Read the model definition and answer for the solid it produces. Units are mm, in the model's axes. A direction names the side the tool comes from. Coordinates: 2 decimals unless noted, no trailing zeros. Loops run counter-clockwise (first coordinate to the right, second up) from the corner with the lowest first, then second, coordinate; pieces in that order, holes last. Notation, with made-up numbers: (-14, 74.25) - (24, 74.25) arc R33 cw to (24, 108.25) - close; hole circle Ø10 at (-12, 71). An arc over 180 degrees is marked (long way). One line per item, written item: value. Start each with the question number.
from build123d import *

# Parameters (mm, degrees)
BOSS_EXTRUDE1_DEPTH = 7.5
FILLET1_R           = 5
SKETCH4_W           = 15
SKETCH4_H           = 20
CUT_EXTRUDE1_DEPTH  = 152.492574085
CUT_EXTRUDE2_DEPTH  = 152.848641751
BOSS_EXTRUDE2_DEPTH = 80
BOSS_EXTRUDE3_START = 5
BOSS_EXTRUDE3_DEPTH = 5
SKETCH9_W           = 12.5
SKETCH9_H           = 20
CUT_EXTRUDE3_DEPTH  = 3
SKETCH10_W          = 2.5
SKETCH10_H          = 200
CUT_EXTRUDE4_DEPTH  = 175.180940404
SKETCH11_R          = 1.85
CUT_EXTRUDE5_DEPTH  = 167.580310961
SKETCH12_R          = 3
SKETCH12_R_2        = 3.25
CUT_EXTRUDE6_DEPTH  = 1
CUT_EXTRUDE7_DEPTH  = 7.5


with BuildPart() as part:
    # Sketch1 → Boss-Extrude1 (new, symmetric)
    with BuildSketch(Plane.XY):
        with BuildLine():
            Line((-7.4, -150), (7.4, -150))
            Line((7.4, -150), (7.4, -100))
            Line((7.4, -100), (15, -100))
            Line((15, -100), (15, 100))
            ThreePointArc((15, 100), (0, 115), (-15, 100))
            Line((-15, 100), (-15, -100))
            Line((-15, -100), (-7.4, -100))
            Line((-7.4, -100), (-7.4, -150))
        make_face()
    extrude(amount=BOSS_EXTRUDE1_DEPTH, both=True)

    # Fillet1
    fillet1_edges = [part.edges().sort_by_distance(p)[0] for p in [
        (7.4, -150, 0),
        (-7.4, -150, 0),
        (15, 0, 7.5),
        (0, 115, 7.5),
        (-15, 0, 7.5),
        (-15, 0, -7.5),
        (0, 115, -7.5),
        (15, 0, -7.5),
    ]]
    fillet(fillet1_edges, radius=FILLET1_R)

    # Sketch4 → Cut-Extrude1 (cut, through all)
    with BuildSketch(Plane.XY.offset(7.5)):
        with Locations((0, -10)):
            Rectangle(SKETCH4_W, SKETCH4_H)
    extrude(amount=-CUT_EXTRUDE1_DEPTH, mode=Mode.SUBTRACT)

    # Sketch5 → Revolve2 (revolve)
    with BuildSketch(Plane.XY):
        with BuildLine():
            Line((-7.5, -10), (-5.5, -10))
            ThreePointArc((-5.5, -10), (-6.085786438, -8.585786438), (-7.5, -8))
            Line((-7.5, -8), (-7.5, -10))
        make_face()
        with BuildLine():
            Line((7.5, -10), (5.5, -10))
            ThreePointArc((5.5, -10), (6.085786438, -8.585786438), (7.5, -8))
            Line((7.5, -8), (7.5, -10))
        make_face()
    revolve(axis=Axis((-21.965922243, -10, 0), (1, 0, 0)))

    # Sketch2 → Cut-Revolve1 (revolve, cut)
    with BuildSketch(Plane.XY):
        with BuildLine():
            Line((-7.4, -138), (-7.4, -140))
            Line((-7.4, -140), (-5.4, -140))
            ThreePointArc((-5.4, -140), (-5.985786438, -138.585786438), (-7.4, -138))
        make_face()
        with BuildLine():
            Line((7.4, -138), (7.4, -140))
            Line((7.4, -140), (5.4, -140))
            ThreePointArc((5.4, -140), (5.985786438, -138.585786438), (7.4, -138))
        make_face()
    revolve(axis=Axis((-23.291382295, -140, 0), (1, 0, 0)), mode=Mode.SUBTRACT)

    # Sketch6 → Cut-Extrude2 (cut, through all)
    with BuildSketch(Plane.ZY.offset(7.4)):
        with BuildLine():
            Line((-7.5, -137.5), (-7.5, -150))
            Line((-7.5, -150), (7.5, -150))
            Line((7.5, -150), (7.5, -137.5))
            ThreePointArc((7.5, -137.5), (0, -145), (-7.5, -137.5))
        make_face()
    extrude(amount=-CUT_EXTRUDE2_DEPTH, mode=Mode.SUBTRACT)

    # Sketch3 → Boss-Extrude2 (add)
    with BuildSketch(Plane(origin=(0, 0, 0), x_dir=(0, 0, -1), z_dir=(1, 0, 0))):
        with BuildLine():
            Line((17, -109.987492178), (17, -104.987492178))
            ThreePointArc((17, -104.987492178), (12.403805922, -103.083686255), (10.5, -98.487492178))
            Line((10.5, -98.487492178), (10.5, 100))
            Line((10.5, 100), (7.5, 100))
            Line((7.5, 100), (7.5, -100))
            ThreePointArc((7.5, -100), (10.254311627, -106.892024376), (17, -109.987492178))
        make_face()
    extrude(amount=BOSS_EXTRUDE2_DEPTH)

    # Sketch7 → Boss-Extrude3 (add)
    with BuildSketch(Plane.ZY.offset(BOSS_EXTRUDE3_START)):
        with BuildLine():
            Line((-10.5, 100), (-7.5, 100))
            Line((-7.5, 100), (-7.5, 0))
            Line((-7.5, 0), (-7.5, -20))
            Line((-7.5, -20), (-7.5, -100))
            ThreePointArc((-7.5, -100), (-10.254311627, -106.892024376), (-17, -109.987492178))
            Line((-17, -109.987492178), (-17, -104.987492178))
            ThreePointArc((-17, -104.987492178), (-12.403805922, -103.083686255), (-10.5, -98.487492178))
            Line((-10.5, -98.487492178), (-10.5, 100))
        make_face()
    extrude(amount=-BOSS_EXTRUDE3_DEPTH)

    # Sketch9 → Cut-Extrude3 (cut)
    with BuildSketch(Plane(origin=(0, 0, -10.5), x_dir=(-1, 0, 0), z_dir=(0, 0, -1))):
        with Locations((-1.25, -10)):
            Rectangle(SKETCH9_W, SKETCH9_H)
    extrude(amount=-CUT_EXTRUDE3_DEPTH, mode=Mode.SUBTRACT)

    # Sketch10 → Cut-Extrude4 (cut, through all)
    with BuildSketch(Plane.ZY.offset(15)):
        with Locations((6.25, 0)):
            Rectangle(SKETCH10_W, SKETCH10_H)
    extrude(amount=-CUT_EXTRUDE4_DEPTH, mode=Mode.SUBTRACT)

    # Sketch11 → Cut-Extrude5 (cut, through all)
    with BuildSketch(Plane(origin=(0, 0, -10.5), x_dir=(-1, 0, 0), z_dir=(0, 0, -1))):
        with Locations(Location((-38, 83.512507822, 0), (0, 0, 90))):
            Circle(SKETCH11_R)
        with Locations(Location((-38, 51.512507822, 0), (0, 0, 90))):
            Circle(SKETCH11_R)
        with Locations(Location((-70, 83.512507822, 0), (0, 0, 90))):
            Circle(SKETCH11_R)
        with Locations(Location((-70, 51.512507822, 0), (0, 0, 90))):
            Circle(SKETCH11_R)
        Polygon((-46.5, 87.012507822), (-61.5, 87.012507822), (-73.5, 75.012507822), (-73.5, 60.012507822), (-61.5, 48.012507822), (-46.5, 48.012507822), (-34.5, 60.012507822), (-34.5, 75.012507822), align=None)
    extrude(amount=-CUT_EXTRUDE5_DEPTH, mode=Mode.SUBTRACT)

    # Sketch12 → Cut-Extrude6 (cut)
    with BuildSketch(Plane(origin=(0, 0, -10.5), x_dir=(-1, 0, 0), z_dir=(0, 0, -1))):
        with Locations(Location((-38, 83.512507822, 0), (0, 0, 90))):
            Circle(SKETCH12_R)
        with Locations(Location((-70, 83.512507822, 0), (0, 0, 90))):
            Circle(SKETCH12_R)
        with Locations(Location((-70, 51.512507822, 0), (0, 0, 90))):
            Circle(SKETCH12_R)
        with Locations(Location((-38, 51.512507822, 0), (0, 0, 90))):
            Circle(SKETCH12_R_2)
    extrude(amount=-CUT_EXTRUDE6_DEPTH, mode=Mode.SUBTRACT)

    # Sketch13 → Cut-Extrude7 (cut, symmetric)
    with BuildSketch(Plane(origin=(0, 0, 0), x_dir=(0, 0, -1), z_dir=(1, 0, 0))):
        Polygon((2.75, 0), (-5, 0), (-5, 12), align=None)
    extrude(amount=CUT_EXTRUDE7_DEPTH, both=True, mode=Mode.SUBTRACT)


solid = part.part
1) Section B-B, the plane y = -94.5 is taken. Determine the outline of the cut face in (x, z), and give its area (3 significant figures).
2) Section A-A, the plane x = 0 is taken. Determine the outline of the cut face in (y, z), and give its area (3 significant figures).
3) Straight lines are drawn through the part: L1, parallel to Z at x = 14, y = 25; L2, parallel to X at y = -46.5, z = -2.5; L3, parallel to Z at x = 26.5, y = -52.5. For each, find the intervals that lie inside material, in ascending order.
4) Section C-C, the plane x = 30.5 is taken. Determine the outline of the cut face in (y, z).
5) Determine the mould class of faces 6 (the flat face through (0, 104, 7.5)), 7 (the cylindrical face through (-13.57, -1.4, -6)), 8 (the flat face through (7.4, -123, 0)), 9 (the flat face through (-7.5, -8, -1)) for opening direction X: released by +X, released by -X, zero draft, split by the parting line, or undercut.
6) Flat-ended cylindrical pins translate along their axes: P1, Ø4, axis at y = 51, z = -3, coming from the +X side; P2, Ø2, axis at x = 15, z = -11.5, coming from the -Y side; P3, Ø3.5, axis at x = 25.5, z = -9, coming from the +Y side; P4, Ø2, axis at x = 38, y = 51.51, coming from the +Z side. Find the tip coordinate at first contact, or state that the pin passes through.
7) For faces 1 (the flat face through (15, -1, 0)), 2 (the flat face through (11, -100, -1)), 3 (the flat face through (0, -20, -3)), 4 (the cylindrical face through (68.175, 81.132, -10.007)), 5 (the flat face through (-5, -65, -8)), determine the directions among +Z, -Z, +X, -X, +Y, -Y from which every point of the face is accessible in a straight line to the end or side of a thin tool.
Answer below:
1. outline: (-15, -2.5) arc R5 ccw to (-10, -7.5) - (-5, -7.5) - (-5, -10.5) - (80, -10.5) - (80, -7.5) - (10, -7.5) arc R5 ccw to (15, -2.5) - (15, 2.5) arc R5 ccw to (14.33, 5) - (-14.33, 5) arc R5 ccw to (-15, 2.5) - close
1. area: 618 mm2
2. outline: (-137.5, -7.5) - (-100, -7.5) arc R10 ccw to (-109.99, -17) - (-104.99, -17) arc R6.5 cw to (-98.49, -10.5) - (-20, -10.5) - (-20, 5) - (-100, 5) - (-100, 7.5) - (-137.5, 7.5) arc R7.5 ccw to start; (0, -10.5) - (100, -10.5) - (100, -7.5) - (110, -7.5) arc R5 ccw to (115, -2.5) - (115, 2.5) arc R5 ccw to (110, 7.5) - (100, 7.5) - (100, 5) - (12, 5) - (0, -2.75) - close
2. area: 3,660 mm2
3. L1: -10.5 to -7.5, -5.5 to 5
3. L2: -15 to 15
3. L3: -10.5 to -7.5
4. outline: (-109.99, -17) - (-104.99, -17) arc R6.5 cw to (-98.49, -10.5) - (100, -10.5) - (100, -7.5) - (-100, -7.5) arc R10 ccw to start
5. face 6: zero draft
5. face 7: released by -X
5. face 8: released by +X
5. face 9: undercut
6. P1: x = 15
6. P2: y = -108.66
6. P3: y = 100
6. P4: through
7. face 1: +Z, +X, +Y, -Y
7. face 2: +Z, +X, -Y
7. face 3: +Z, -Z
7. face 4: -Z
7. face 5: -Z, -X, +Y, -Y
